Job drawing, mm, ordinate dimensions from the low corner. One solid piece. Give positions to 0.01 mm unless a question says otherwise; leave off trailing zeros. Loops run counter-clockwise (first coordinate to the right, second up) from the corner with the lowest first, then second, coordinate; pieces in that order, holes last. Notation, with made-up numbers: (1, 55) -> (26, 55) arc R31 ccw to (26, 87) -> close; hole circle Ø10 at (82.5, -18). An arc over 180 degrees is marked (long way). Use one line per item in the form item = value.
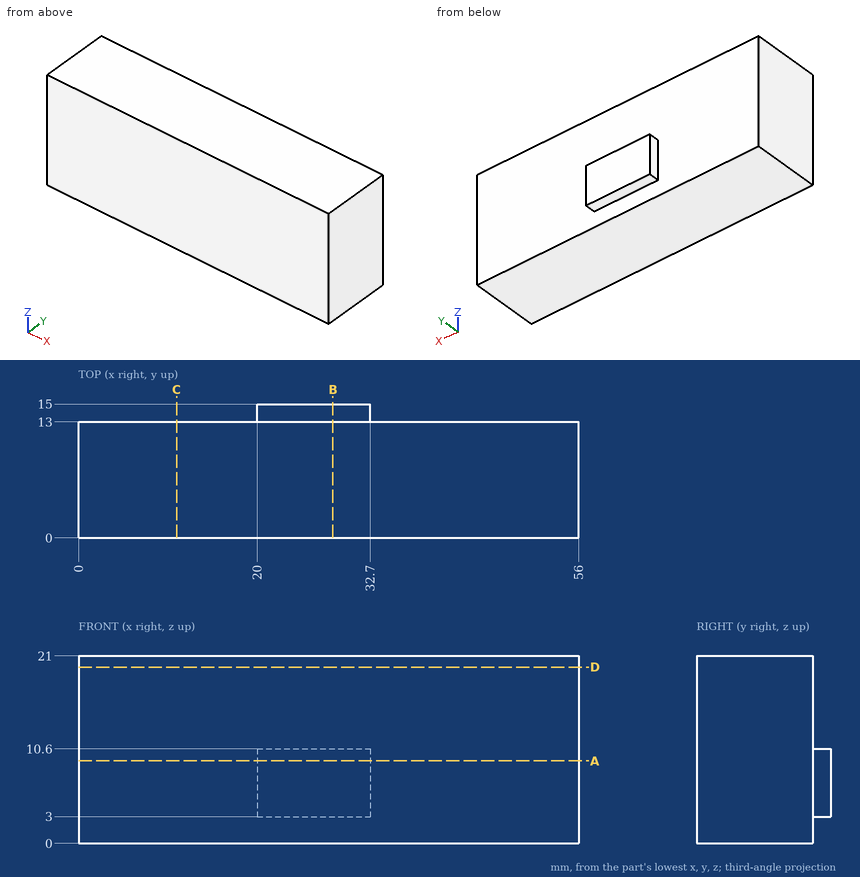
1. Cut at A-A, the plane z = 9.25. Write the cut outline in (x, y), then the cut area to 3 significant figures.
Result sheet:
outline = (0, 0) -> (56, 0) -> (56, 13) -> (32.7, 13) -> (32.7, 15) -> (20, 15) -> (20, 13) -> (0, 13) -> close
area = 753 mm^2
2. Cut at C-C, the plane x = 11. Write the cut outline in (y, z).
Result sheet:
outline = (0, 0) -> (13, 0) -> (13, 21) -> (0, 21) -> close
3. Drill centre line: line 1 (Y direction, x = 46.5, z = 4.75). Where is it in solid material? Low to high.
Result sheet:
line_1 = 0 to 13
4. Drop flat-ended pins along their axis: P1, Ø1.5, axis at y = 7.5, z = 7, coming from the -X side; P2, Ø2, axis at x = 35, z = 4.5, coming from the +Y side; P3, Ø0.6, axis at y = 14, z = 7.5, coming from the +X side. Give the stop position or say it passes through.
Result sheet:
P1 = 0
P2 = 13
P3 = 32.7
5. Cut at B-B, the plane x = 28.5. Write the cut outline in (y, z), then the cut area to 3 significant figures.
Result sheet:
outline = (0, 0) -> (13, 0) -> (13, 3) -> (15, 3) -> (15, 10.6) -> (13, 10.6) -> (13, 21) -> (0, 21) -> close
area = 288 mm^2
6. Cut at D-D, the plane z = 19.75. Write the cut outline in (x, y), then the cut area to 3 significant figures.
Result sheet:
outline = (0, 0) -> (56, 0) -> (56, 13) -> (0, 13) -> close
area = 728 mm^2
